from build123d import *

# Parameters (mm, degrees)
ESQUISSE1_R             = 1.65
BOSS_EXTRU_1_DEPTH      = 11
BOSS_EXTRU_2_REACH      = 35.597
ESQUISSE2_W             = 22
ESQUISSE2_H             = 6.5
ENL_V_MAT_EXTRU_1_DEPTH = 30


with BuildPart() as part:
    # Esquisse1 → Boss.-Extru.1 (new, symmetric)
    with BuildSketch(Plane.XY):
        with BuildLine():
            Line((11.628725406, -24), (16.628725406, -24))
            Line((16.628725406, -24), (16.628725406, -11))
            Line((16.628725406, -11), (15.628725406, -11))
            Line((15.628725406, -11), (3.068517607, 2.794047189))
            ThreePointArc((3.068517607, 2.794047189), (-1.728115101, 3.77307808), (-4.119967472, -0.49836536))
            Line((-4.119967472, -0.49836536), (11.628725406, -24))
        make_face()
        Circle(ESQUISSE1_R, mode=Mode.SUBTRACT)
    extrude(amount=BOSS_EXTRU_1_DEPTH, both=True)

    # Boss.-Extru.2: up to this plane
    boss_extru_2_end = Plane(origin=(-4.119967472, -0.49836536, 11), z_dir=(0.8307275154862657, 0.5566792568562408, 0))
    # Esquisse2 → Boss.-Extru.2 (add, up to the surface)
    with BuildSketch(Plane(origin=(16.628725406, 0, 0), x_dir=(0, 0, -1), z_dir=(1, 0, 0)), mode=Mode.PRIVATE) as boss_extru_2_sk1:
        with BuildLine():
            ThreePointArc((-18.5, -13.75), (-15.848349571, -14.848349571), (-14.75, -17.5))
            Line((-14.75, -17.5), (-11, -17.5))
            Line((-11, -17.5), (-11, -11))
            Line((-11, -11), (-18.5, -11))
            Line((-18.5, -11), (-18.5, -13.75))
        make_face()
    boss_extru_2_tool1 = split(extrude(boss_extru_2_sk1.sketch, amount=-BOSS_EXTRU_2_REACH, mode=Mode.PRIVATE), bisect_by=boss_extru_2_end, keep=Keep.BOTH, mode=Mode.PRIVATE)
    add(boss_extru_2_tool1.solids().sort_by_distance((16.628725, -13.764206, 14.117746))[0])
    # Esquisse2 → Boss.-Extru.2 (add, up to the surface)
    with BuildSketch(Plane(origin=(16.628725406, 0, 0), x_dir=(0, 0, -1), z_dir=(1, 0, 0)), mode=Mode.PRIVATE) as boss_extru_2_sk2:
        with BuildLine():
            Line((-11, -17.5), (-14.75, -17.5))
            ThreePointArc((-14.75, -17.5), (-15.848349571, -20.151650429), (-18.5, -21.25))
            Line((-18.5, -21.25), (-18.5, -24))
            Line((-18.5, -24), (-11, -24))
            Line((-11, -24), (-11, -17.5))
        make_face()
    boss_extru_2_tool2 = split(extrude(boss_extru_2_sk2.sketch, amount=-BOSS_EXTRU_2_REACH, mode=Mode.PRIVATE), bisect_by=boss_extru_2_end, keep=Keep.BOTH, mode=Mode.PRIVATE)
    add(boss_extru_2_tool2.solids().sort_by_distance((16.628725, -21.235794, 14.117746))[0])
    # Esquisse2 → Boss.-Extru.2 (add, up to the surface)
    with BuildSketch(Plane(origin=(16.628725406, 0, 0), x_dir=(0, 0, -1), z_dir=(1, 0, 0)), mode=Mode.PRIVATE) as boss_extru_2_sk3:
        with BuildLine():
            ThreePointArc((-18.5, -16.5), (-17.792893219, -16.792893219), (-17.5, -17.5))
            Line((-17.5, -17.5), (-14.75, -17.5))
            ThreePointArc((-14.75, -17.5), (-15.848349571, -14.848349571), (-18.5, -13.75))
            Line((-18.5, -13.75), (-18.5, -16.5))
        make_face()
    boss_extru_2_tool3 = split(extrude(boss_extru_2_sk3.sketch, amount=-BOSS_EXTRU_2_REACH, mode=Mode.PRIVATE), bisect_by=boss_extru_2_end, keep=Keep.BOTH, mode=Mode.PRIVATE)
    add(boss_extru_2_tool3.solids().sort_by_distance((16.628725, -15.8191, 16.8191))[0])
    # Esquisse2 → Boss.-Extru.2 (add, up to the surface)
    with BuildSketch(Plane(origin=(16.628725406, 0, 0), x_dir=(0, 0, -1), z_dir=(1, 0, 0)), mode=Mode.PRIVATE) as boss_extru_2_sk4:
        with BuildLine():
            Line((-14.75, -17.5), (-17.5, -17.5))
            ThreePointArc((-17.5, -17.5), (-17.792893219, -18.207106781), (-18.5, -18.5))
            Line((-18.5, -18.5), (-18.5, -21.25))
            ThreePointArc((-18.5, -21.25), (-15.848349571, -20.151650429), (-14.75, -17.5))
        make_face()
    boss_extru_2_tool4 = split(extrude(boss_extru_2_sk4.sketch, amount=-BOSS_EXTRU_2_REACH, mode=Mode.PRIVATE), bisect_by=boss_extru_2_end, keep=Keep.BOTH, mode=Mode.PRIVATE)
    add(boss_extru_2_tool4.solids().sort_by_distance((16.628725, -19.1809, 16.8191))[0])
    # Esquisse2 → Boss.-Extru.2 (add, up to the surface)
    with BuildSketch(Plane(origin=(16.628725406, 0, 0), x_dir=(0, 0, -1), z_dir=(1, 0, 0)), mode=Mode.PRIVATE) as boss_extru_2_sk5:
        with BuildLine():
            ThreePointArc((-18.5, -16.5), (-17.792893219, -16.792893219), (-17.5, -17.5))
            Line((-17.5, -17.5), (-14.75, -17.5))
            ThreePointArc((-14.75, -17.5), (-15.848349571, -14.848349571), (-18.5, -13.75))
            Line((-18.5, -13.75), (-18.5, -16.5))
        make_face()
    boss_extru_2_tool5 = split(extrude(boss_extru_2_sk5.sketch, amount=-BOSS_EXTRU_2_REACH, mode=Mode.PRIVATE), bisect_by=boss_extru_2_end, keep=Keep.BOTH, mode=Mode.PRIVATE)
    add(boss_extru_2_tool5.solids().sort_by_distance((16.628725, -15.8191, 16.8191))[0])
    # Esquisse2 → Boss.-Extru.2 (add, up to the surface)
    with BuildSketch(Plane(origin=(16.628725406, 0, 0), x_dir=(0, 0, -1), z_dir=(1, 0, 0)), mode=Mode.PRIVATE) as boss_extru_2_sk6:
        with BuildLine():
            Line((-14.75, -17.5), (-17.5, -17.5))
            ThreePointArc((-17.5, -17.5), (-17.792893219, -18.207106781), (-18.5, -18.5))
            Line((-18.5, -18.5), (-18.5, -21.25))
            ThreePointArc((-18.5, -21.25), (-15.848349571, -20.151650429), (-14.75, -17.5))
        make_face()
    boss_extru_2_tool6 = split(extrude(boss_extru_2_sk6.sketch, amount=-BOSS_EXTRU_2_REACH, mode=Mode.PRIVATE), bisect_by=boss_extru_2_end, keep=Keep.BOTH, mode=Mode.PRIVATE)
    add(boss_extru_2_tool6.solids().sort_by_distance((16.628725, -19.1809, 16.8191))[0])
    # Esquisse2 → Boss.-Extru.2 (add, up to the surface)
    with BuildSketch(Plane(origin=(16.628725406, 0, 0), x_dir=(0, 0, -1), z_dir=(1, 0, 0)), mode=Mode.PRIVATE) as boss_extru_2_sk7:
        with BuildLine():
            ThreePointArc((-18.5, -18.5), (-19.5, -17.5), (-18.5, -16.5))
            Line((-18.5, -16.5), (-18.5, -13.75))
            ThreePointArc((-18.5, -13.75), (-22.25, -17.5), (-18.5, -21.25))
            Line((-18.5, -21.25), (-18.5, -18.5))
        make_face()
    boss_extru_2_tool7 = split(extrude(boss_extru_2_sk7.sketch, amount=-BOSS_EXTRU_2_REACH, mode=Mode.PRIVATE), bisect_by=boss_extru_2_end, keep=Keep.BOTH, mode=Mode.PRIVATE)
    add(boss_extru_2_tool7.solids().sort_by_distance((16.628725, -17.5, 20.1809))[0])
    # Esquisse2 → Boss.-Extru.2 (add, up to the surface)
    with BuildSketch(Plane(origin=(16.628725406, 0, 0), x_dir=(0, 0, -1), z_dir=(1, 0, 0)), mode=Mode.PRIVATE) as boss_extru_2_sk8:
        with Locations((0, -14.25)):
            Rectangle(ESQUISSE2_W, ESQUISSE2_H)
    boss_extru_2_tool8 = split(extrude(boss_extru_2_sk8.sketch, amount=-BOSS_EXTRU_2_REACH, mode=Mode.PRIVATE), bisect_by=boss_extru_2_end, keep=Keep.BOTH, mode=Mode.PRIVATE)
    add(boss_extru_2_tool8.solids().sort_by_distance((16.628725, -14.25, 0))[0])
    # Esquisse2 → Boss.-Extru.2 (add, up to the surface)
    with BuildSketch(Plane(origin=(16.628725406, 0, 0), x_dir=(0, 0, -1), z_dir=(1, 0, 0)), mode=Mode.PRIVATE) as boss_extru_2_sk9:
        with Locations((0, -20.75)):
            Rectangle(ESQUISSE2_W, ESQUISSE2_H)
    boss_extru_2_tool9 = split(extrude(boss_extru_2_sk9.sketch, amount=-BOSS_EXTRU_2_REACH, mode=Mode.PRIVATE), bisect_by=boss_extru_2_end, keep=Keep.BOTH, mode=Mode.PRIVATE)
    add(boss_extru_2_tool9.solids().sort_by_distance((16.628725, -20.75, 0))[0])
    # Esquisse2 → Boss.-Extru.2 (add, up to the surface)
    with BuildSketch(Plane(origin=(16.628725406, 0, 0), x_dir=(0, 0, -1), z_dir=(1, 0, 0)), mode=Mode.PRIVATE) as boss_extru_2_sk10:
        with BuildLine():
            Line((11, -11), (11, -17.5))
            Line((11, -17.5), (14.75, -17.5))
            ThreePointArc((14.75, -17.5), (15.848349571, -14.848349571), (18.5, -13.75))
            Line((18.5, -13.75), (18.5, -11))
            Line((18.5, -11), (11, -11))
        make_face()
    boss_extru_2_tool10 = split(extrude(boss_extru_2_sk10.sketch, amount=-BOSS_EXTRU_2_REACH, mode=Mode.PRIVATE), bisect_by=boss_extru_2_end, keep=Keep.BOTH, mode=Mode.PRIVATE)
    add(boss_extru_2_tool10.solids().sort_by_distance((16.628725, -13.764206, -14.117746))[0])
    # Esquisse2 → Boss.-Extru.2 (add, up to the surface)
    with BuildSketch(Plane(origin=(16.628725406, 0, 0), x_dir=(0, 0, -1), z_dir=(1, 0, 0)), mode=Mode.PRIVATE) as boss_extru_2_sk11:
        with BuildLine():
            Line((14.75, -17.5), (11, -17.5))
            Line((11, -17.5), (11, -24))
            Line((11, -24), (18.5, -24))
            Line((18.5, -24), (18.5, -21.25))
            ThreePointArc((18.5, -21.25), (15.848349571, -20.151650429), (14.75, -17.5))
        make_face()
    boss_extru_2_tool11 = split(extrude(boss_extru_2_sk11.sketch, amount=-BOSS_EXTRU_2_REACH, mode=Mode.PRIVATE), bisect_by=boss_extru_2_end, keep=Keep.BOTH, mode=Mode.PRIVATE)
    add(boss_extru_2_tool11.solids().sort_by_distance((16.628725, -21.235794, -14.117746))[0])
    # Esquisse2 → Boss.-Extru.2 (add, up to the surface)
    with BuildSketch(Plane(origin=(16.628725406, 0, 0), x_dir=(0, 0, -1), z_dir=(1, 0, 0)), mode=Mode.PRIVATE) as boss_extru_2_sk12:
        with BuildLine():
            ThreePointArc((18.5, -13.75), (15.848349571, -14.848349571), (14.75, -17.5))
            Line((14.75, -17.5), (17.5, -17.5))
            ThreePointArc((17.5, -17.5), (17.792893219, -16.792893219), (18.5, -16.5))
            Line((18.5, -16.5), (18.5, -13.75))
        make_face()
    boss_extru_2_tool12 = split(extrude(boss_extru_2_sk12.sketch, amount=-BOSS_EXTRU_2_REACH, mode=Mode.PRIVATE), bisect_by=boss_extru_2_end, keep=Keep.BOTH, mode=Mode.PRIVATE)
    add(boss_extru_2_tool12.solids().sort_by_distance((16.628725, -15.8191, -16.8191))[0])
    # Esquisse2 → Boss.-Extru.2 (add, up to the surface)
    with BuildSketch(Plane(origin=(16.628725406, 0, 0), x_dir=(0, 0, -1), z_dir=(1, 0, 0)), mode=Mode.PRIVATE) as boss_extru_2_sk13:
        with BuildLine():
            Line((17.5, -17.5), (14.75, -17.5))
            ThreePointArc((14.75, -17.5), (15.848349571, -20.151650429), (18.5, -21.25))
            Line((18.5, -21.25), (18.5, -18.5))
            ThreePointArc((18.5, -18.5), (17.792893219, -18.207106781), (17.5, -17.5))
        make_face()
    boss_extru_2_tool13 = split(extrude(boss_extru_2_sk13.sketch, amount=-BOSS_EXTRU_2_REACH, mode=Mode.PRIVATE), bisect_by=boss_extru_2_end, keep=Keep.BOTH, mode=Mode.PRIVATE)
    add(boss_extru_2_tool13.solids().sort_by_distance((16.628725, -19.1809, -16.8191))[0])
    # Esquisse2 → Boss.-Extru.2 (add, up to the surface)
    with BuildSketch(Plane(origin=(16.628725406, 0, 0), x_dir=(0, 0, -1), z_dir=(1, 0, 0)), mode=Mode.PRIVATE) as boss_extru_2_sk14:
        with BuildLine():
            ThreePointArc((18.5, -13.75), (15.848349571, -14.848349571), (14.75, -17.5))
            Line((14.75, -17.5), (17.5, -17.5))
            ThreePointArc((17.5, -17.5), (17.792893219, -16.792893219), (18.5, -16.5))
            Line((18.5, -16.5), (18.5, -13.75))
        make_face()
    boss_extru_2_tool14 = split(extrude(boss_extru_2_sk14.sketch, amount=-BOSS_EXTRU_2_REACH, mode=Mode.PRIVATE), bisect_by=boss_extru_2_end, keep=Keep.BOTH, mode=Mode.PRIVATE)
    add(boss_extru_2_tool14.solids().sort_by_distance((16.628725, -15.8191, -16.8191))[0])
    # Esquisse2 → Boss.-Extru.2 (add, up to the surface)
    with BuildSketch(Plane(origin=(16.628725406, 0, 0), x_dir=(0, 0, -1), z_dir=(1, 0, 0)), mode=Mode.PRIVATE) as boss_extru_2_sk15:
        with BuildLine():
            Line((17.5, -17.5), (14.75, -17.5))
            ThreePointArc((14.75, -17.5), (15.848349571, -20.151650429), (18.5, -21.25))
            Line((18.5, -21.25), (18.5, -18.5))
            ThreePointArc((18.5, -18.5), (17.792893219, -18.207106781), (17.5, -17.5))
        make_face()
    boss_extru_2_tool15 = split(extrude(boss_extru_2_sk15.sketch, amount=-BOSS_EXTRU_2_REACH, mode=Mode.PRIVATE), bisect_by=boss_extru_2_end, keep=Keep.BOTH, mode=Mode.PRIVATE)
    add(boss_extru_2_tool15.solids().sort_by_distance((16.628725, -19.1809, -16.8191))[0])
    # Esquisse2 → Boss.-Extru.2 (add, up to the surface)
    with BuildSketch(Plane(origin=(16.628725406, 0, 0), x_dir=(0, 0, -1), z_dir=(1, 0, 0)), mode=Mode.PRIVATE) as boss_extru_2_sk16:
        with BuildLine():
            ThreePointArc((22.25, -17.5), (21.151650429, -14.848349571), (18.5, -13.75))
            Line((18.5, -13.75), (18.5, -16.5))
            ThreePointArc((18.5, -16.5), (19.207106781, -16.792893219), (19.5, -17.5))
            ThreePointArc((19.5, -17.5), (19.207106781, -18.207106781), (18.5, -18.5))
            Line((18.5, -18.5), (18.5, -21.25))
            ThreePointArc((18.5, -21.25), (21.151650429, -20.151650429), (22.25, -17.5))
        make_face()
    boss_extru_2_tool16 = split(extrude(boss_extru_2_sk16.sketch, amount=-BOSS_EXTRU_2_REACH, mode=Mode.PRIVATE), bisect_by=boss_extru_2_end, keep=Keep.BOTH, mode=Mode.PRIVATE)
    add(boss_extru_2_tool16.solids().sort_by_distance((16.628725, -17.5, -20.1809))[0])

    # Esquisse3 → Enl_v. mat.-Extru.1 (cut)
    with BuildSketch(Plane(origin=(16.628725406, 0, 0), x_dir=(0, 0, -1), z_dir=(1, 0, 0))):
        Polygon((-6, 4.15), (-6, -4.35), (-11, -11), (-11, 4.15), align=None)
    extrude(amount=-ENL_V_MAT_EXTRU_1_DEPTH, mode=Mode.SUBTRACT)


solid = part.part
Geometry: final body of the model. Coordinates: model frame, mm. A direction names the side the tool comes from. Round coordinates to 2 decimals unless told otherwise and drop trailing zeros. Loops run counter-clockwise (first coordinate to the right, second up) from the corner with the lowest first, then second, coordinate; pieces in that order, holes last.
Q1. Section A-A on y = 0. Return loops of the section in (x, z), plus the area to 3 significant figures.
Q2. Material intervals for L1, parallel to Y at x = 0, z = 1; L2, parallel to Z at x = 2.25, y = -2.25; L3, parallel to Z at x = 15, y = -12, sorted ascending.
Q3. Section C-C on x = 12.75. Return loops of the section in (y, z), plus the area to 3 significant figures.
Q4. Pull-direction query (X, two-part tool) for faces 5 (the cylindrical face through (-1.661, 3.803, -2.381)), 6 (the flat face through (10, -12, 18.5)), 7 (the cylindrical face through (-1.216, 1.115, -2.619)); classes: released by +X, released by -X, zero draft, split by the parting line, or undercut.
Q5. Pin query (flat end, axial travel): P1, Ø1, axis at x = 9, y = -13, coming from the +Z side; P2, Ø9.5, axis at x = 2.5, y = 0, coming from the +Z side; P3, Ø8, axis at x = 5, y = 1, coming from the +Z side; P4, Ø2.5, axis at x = 0, y = 0, coming from the +Z side. Return the tip coordinate at first contact, or that it passes through.
Q6. Access query for faces 1 (the flat face through (14, -23, -18.5)), 2 (the flat face through (3, -5, -11)), 3 (the flat face through (16, -11, 0)), 4 (the flat face through (14, -23, 18.5)). Directions: +Z, -Z, +X, -X, +Y, -Y. A direction counts if a zero-diameter tool reaches every point of the face in a straight line with its end or side. Return the directions, or none.
Q7. Section D-D on z = 15.5. Return loops of the section in (x, y).
Q8. Section B-B on x = 0. Return loops of the section in (y, z).
Evaluation:
1. outline: (-4.15, -11) - (-1.65, -11) - (-1.65, 6) - (-4.15, 6) - close; (1.65, -11) - (5.61, -11) - (5.61, 6) - (1.65, 6) - close
1. area: 110 mm2
2. L1: y = -6.65 to -1.65, 1.65 to 4.15
2. L2: z = -11 to 6
2. L3: z = -18.5 to 18.5
3. outline: (-24, -18.5) - (-21.25, -18.5) arc R3.75 ccw to (-13.75, -18.5) - (-11, -18.5) - (-11, -11) - (-7.84, -11) - (-7.84, 8.62) - (-11, 11) - (-11, 18.5) - (-13.75, 18.5) arc R3.75 ccw to (-21.25, 18.5) - (-24, 18.5) - close; hole circle Ø2 at (-17.5, -18.5); hole circle Ø2 at (-17.5, 18.5)
3. area: 585 mm2
4. face 5: split by the parting line
4. face 6: zero draft
4. face 7: undercut
5. P1: stops at z = 18.5
5. P2: stops at z = 6.3
5. P3: stops at z = 6
5. P4: passes through
6. face 1: -Z, +X, -X, -Y
6. face 2: -Z, +X, -X, +Y
6. face 3: +X, +Y
6. face 4: +Z, +X, -X, -Y
7. outline: (2.92, -11) - (11.63, -24) - (16.63, -24) - (16.63, -11) - close
8. outline: (-6.65, -11) - (-1.65, -11) - (-1.65, 6) - (-4.35, 6) - (-6.65, 7.73) - close; (1.65, -11) - (4.15, -11) - (4.15, 6) - (1.65, 6) - close
